The figure shows three views and two pictorial views of one solid part (mm, origin at its lowest corner). Answer the questions. A direction names the side the tool comes from. Coordinates: 2 decimals unless noted, no trailing zeros. Loops run counter-clockwise (first coordinate to the right, second up) from the corner with the lowest first, then second, coordinate; pieces in that order, holes last. Notation, with made-up numbers: M -30,53.5 L 24,53.5 A13 ccw 24,60.5 Z; hole C 52,-2.75 d6. An arc over 180 degrees is marked long. Answer as a JSON object with one key per item and string values. Group by question number.
1. Determine the mould class of the marked faces 1, 2, 3 and 4 for opening direction Y: released by +Y, released by -Y, zero draft, split by the parting line, or undercut.
2. A cutting plane is placed at D-D on z = 9. Give the vertices of the cut face in (x, y).
3. Straight lines are drawn through the part: L1, parallel to Y at x = 7.5, z = 16; L2, parallel to Y at x = 10.5, z = 3; L3, parallel to X at y = 14.25, z = 8.75. For each, find the intervals that lie inside material, in ascending order.
4. A cutting plane is placed at B-B on z = 15.5. Give the vertices of the cut face in (x, y), and give its area (3 significant figures).
5. A cutting plane is placed at A-A on x = 9. Give the vertices of the cut face in (y, z).
6. For the marked faces 5 and 6, determine the directions among +Z, -Z, +X, -X, +Y, -Y from which every point of the face is accessible in a straight line to the end or side of a thin tool.
7. Given pin 1 (8 mm diameter, centred on y = 2, z = 15, fed in from +X); pin 2 (1.5 mm diameter, centred on x = 9.5, y = 5.5, fed in from +Z); pin 3 (6 mm diameter, centred on y = 3, z = 14, fed in from +X), each flat-ended and moving along its own axis, determine where each tip first touches the part or whether it passes through.
8. A cutting plane is placed at C-C on x = 16. Give the vertices of the cut face in (y, z).
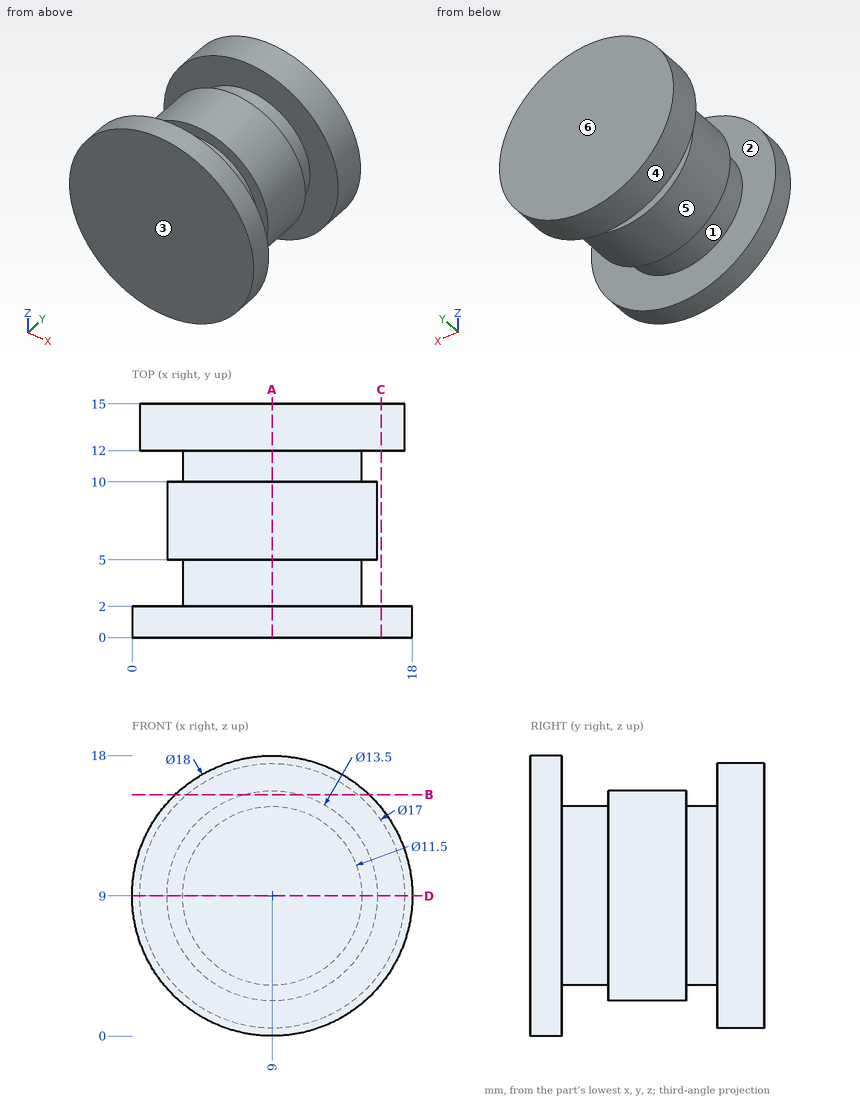
From the geometry:
{
 "1": {"face 1": "undercut", "face 2": "undercut", "face 3": "released by -Y", "face 4": "zero draft"},
 "2": {"outline": "M 0,0 L 18,0 L 18,2 L 14.75,2 L 14.75,5 L 15.75,5 L 15.75,10 L 14.75,10 L 14.75,12 L 17.5,12 L 17.5,15 L 0.5,15 L 0.5,12 L 3.25,12 L 3.25,10 L 2.25,10 L 2.25,5 L 3.25,5 L 3.25,2 L 0,2 Z"},
 "3": {"L1": "y = 0 to 2, 12 to 15", "L2": "y = 0 to 2, 5 to 10, 12 to 15", "L3": "x = 0.5 to 17.5"},
 "4": {"outline": "M 2.78,0 L 15.22,0 L 15.22,2 L 2.78,2 Z; M 3.52,12 L 14.48,12 L 14.48,15 L 3.52,15 Z; M 7.18,5 L 10.82,5 L 10.82,10 L 7.18,10 Z", "area": "76.0 mm²"},
 "5": {"outline": "M 0,0 L 2,0 L 2,3.25 L 5,3.25 L 5,2.25 L 10,2.25 L 10,3.25 L 12,3.25 L 12,0.5 L 15,0.5 L 15,17.5 L 12,17.5 L 12,14.75 L 10,14.75 L 10,15.75 L 5,15.75 L 5,14.75 L 2,14.75 L 2,18 L 0,18 Z"},
 "6": {"face 5": "none", "face 6": "+Z, -Z, +X, -X, +Y"},
 "7": {"pin 1": "stops at x = 17.77", "pin 2": "stops at z = 15.75", "pin 3": "stops at x = 17.73"},
 "8": {"outline": "M 0,3.34 L 2,3.34 L 2,14.66 L 0,14.66 Z; M 12,4.18 L 15,4.18 L 15,13.82 L 12,13.82 Z"}
}
